Part model, mm, in its own coordinate system. A direction names the side the tool comes from. Give positions to 0.01 mm unless a question says otherwise; leave off trailing zeros. Answer as a JSON object with one key per item and string values. Group by question number.
```python
from build123d import *

# Parameters (mm, degrees)
F0_W     = 8
F0_H     = 30
F1_DEPTH = 57
F2_DEPTH = 15
F4_DEPTH = 8


with BuildPart() as f1:
    # F0 (on Top) → F1 (new body)
    with BuildSketch(Plane.XY):
        Rectangle(F0_W, F0_H)
    extrude(amount=F1_DEPTH)

    # F2 (add): a face of the model
    f2_faces = [f1.faces().sort_by_distance(p)[0] for p in [
        (0, 0, 0),
    ]]
    extrude(f2_faces, amount=F2_DEPTH)

    # F3 (on face) → F4 (cut, through all)
    with BuildSketch(Plane(origin=(-4, 0, 0), x_dir=(0, -1, 0), z_dir=(-1, 0, 0))):
        with BuildLine():
            Line((15, 57), (-12, 57))
            Line((-12, 57), (-12, 55.4652698338))
            add(Edge.make_bspline(
                [(-12, 55.4652698338), (4.7257277183, 36.0407754779), (-9.3587208539, 3.8601619937), (-12, -5)],
                knots=[0, 0, 0, 0, 60.4652698338, 60.4652698338, 60.4652698338, 60.4652698338], degree=3))
            Line((-12, -5), (-12, -15))
            Line((-12, -15), (15, -15))
            Line((15, -15), (15, 57))
        make_face()
        with BuildLine():
            add(Edge.make_bspline(
                [(-15, 55.4652698338), (1.0521842632, 33.6701404303), (-12.6800062135, 5.2046555839), (-15, -5)],
                knots=[0, 0, 0, 0, 60.4652698338, 60.4652698338, 60.4652698338, 60.4652698338], degree=3))
            Line((-15, 55.4652698338), (-15, -5))
        make_face()
    extrude(amount=-F4_DEPTH, mode=Mode.SUBTRACT)


solid = f1.part
```
1) Drop flat-ended pins along their axis: P1, Ø1, axis at x = -3, z = 43.5, coming from the +Y side; P2, Ø0.5, axis at x = -1.5, z = 56, coming from the -Y side; P3, Ø4, axis at x = 2, z = 45, coming from the +Y side. Give the stop position or say it passes through.
2) Drill centre lines: line 1 along Y through (x, z) = (1.5, -11); line 2 along Y through (x, z) = (-0.25, 39.5). Where is each one in solid material? Low to high. Write a range as from..to.
3) Which spindle directions (+Z, -Z, +X, -X, +Y, -Y) get a long thin tool onto all of the face, cutting with end or side? Do faces 1 (the flat face through (0, 12, 56)), 2 (the flat face through (0, 12, -10)), 3 (the flat face through (0, 15, -10)). Say none if no direction does.
Checks:
{
 "1": {"P1": "y = 9.23", "P2": "y = 12", "P3": "y = 10.28"},
 "2": {"line 1": "12..15", "line 2": "4.65..8.12"},
 "3": {"face 1": "+Z, +X, -X, -Y", "face 2": "-Z, +X, -X, -Y", "face 3": "+Z, -Z, +X, -X, +Y"}
}
